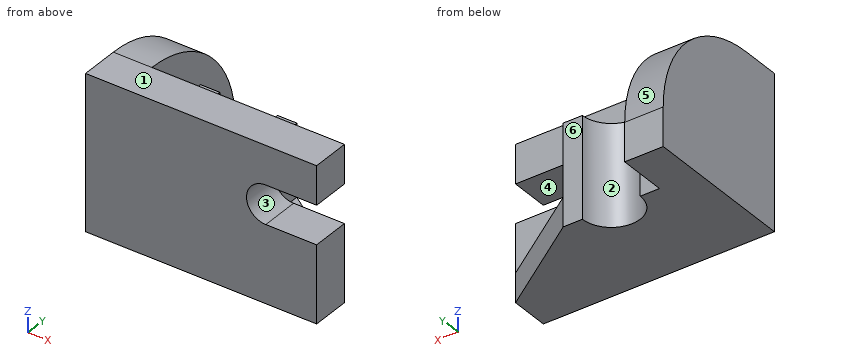
```python
from build123d import *

# Parameters (mm, degrees)
BOSS_EXTRUDE1_DEPTH = 40.64
BOSS_EXTRUDE2_DEPTH = 121.92
BOSS_EXTRUDE3_DEPTH = 71.12
CHAMFER1_SIZE       = 71.12
CHAMFER1_SIZE2      = 101.6
FILLET1_R           = 121.92
CUT_EXTRUDE1_DEPTH  = 106.68


with BuildPart() as part:
    # Sketch1 → Boss-Extrude1 (new body)
    with BuildSketch(Plane(origin=(0, 0, 0), x_dir=(1, 0, 0), z_dir=(0, 1, 0))):
        with BuildLine():
            Line((186.601289805, 121.92), (-57.238710195, 121.92))
            Line((-57.238710195, 121.92), (-57.238710195, -40.64))
            Line((-57.238710195, -40.64), (186.601289805, -40.64))
            Line((186.601289805, -40.64), (186.601289805, 0))
            Line((186.601289805, 0), (132.948481924, 0))
            ThreePointArc((132.948481924, 0), (112.628481924, 20.32), (132.948481924, 40.64))
            Line((132.948481924, 40.64), (186.601289805, 40.64))
            Line((186.601289805, 40.64), (186.601289805, 121.92))
        make_face()
    extrude(amount=BOSS_EXTRUDE1_DEPTH)

    # Sketch2 → Boss-Extrude2 (add)
    with BuildSketch(Plane(origin=(0, 40.64, 0), x_dir=(1, 0, 0), z_dir=(0, 1, 0))):
        Polygon((-16.598710195, 15.24), (-16.598710195, 121.92), (-57.238710195, 121.92), (-57.238710195, -40.64), (-16.598710195, -40.64), align=None)
    extrude(amount=BOSS_EXTRUDE2_DEPTH)

    # Sketch2<4> → Boss-Extrude3 (add)
    with BuildSketch(Plane(origin=(0, 40.64, 0), x_dir=(1, 0, 0), z_dir=(0, 1, 0))):
        Polygon((-16.598710195, 15.24), (85.001289805, 15.24), (85.001289805, 91.44), (186.601289805, 91.44), (186.601289805, 121.92), (-16.598710195, 121.92), align=None)
    extrude(amount=BOSS_EXTRUDE3_DEPTH)

    # Chamfer1
    chamfer1_edges = [part.edges().sort_by_distance(p)[0] for p in [
        (186.601289805, 111.76, -106.68),
    ]]
    chamfer1_side = [part.faces().sort_by_distance(p)[0] for p in [
        (186.601289805, 20.32, -42.021909404),
    ]]
    chamfer(chamfer1_edges, length=CHAMFER1_SIZE, length2=CHAMFER1_SIZE2, reference=chamfer1_side[0])

    # Fillet1
    fillet1_edges = [part.edges().sort_by_distance(p)[0] for p in [
        (-36.918710195, 162.56, 40.64),
    ]]
    fillet(fillet1_edges, radius=FILLET1_R)

    # Sketch3 → Cut-Extrude1 (cut)
    with BuildSketch(Plane.XY.offset(-15.24)):
        with BuildLine():
            Line((64.681289805, 111.76), (3.721289805, 111.76))
            ThreePointArc((3.721289805, 111.76), (34.201289805, 81.28), (64.681289805, 111.76))
        make_face()
    extrude(amount=-CUT_EXTRUDE1_DEPTH, mode=Mode.SUBTRACT)


solid = part.part
```
Can you work these out from the model? Positions are in its coordinate system, mm. Face numbers are marked on the shaded views. A direction names the side the tool comes from. Round coordinates to 2 decimals unless told otherwise and drop trailing zeros. Loops run counter-clockwise (first coordinate to the right, second up) from the corner with the lowest first, then second, coordinate; pieces in that order, holes last. Notation, with made-up numbers: (-13.5, 19) -> (6.5, 19) arc R25 ccw to (6.5, 33) -> close; hole circle Ø7 at (14, -5.75). An arc over 180 degrees is marked (long way). One line per item, written item: value. Start each with the question number.
1. If we section it at C-C, the plane x = 118.5: Write out the boundary of the cut face in (y, z).
2. If we section it at B-B, the plane y = 108: Write out the boundary of the cut face in (x, z).
3. For the marked faces 4, 5 and 6, which set-ups out of +Z, -Z, +X, -X, +Y, -Y let a thin tool reach every point of the face, with its end or its side?
4. For pin 1 (12 mm diameter, centred on y = 50, z = -20, fed in from +X); pin 2 (6 mm diameter, centred on x = -6.5, z = -70, fed in from +Y); pin 3 (21.5 mm diameter, centred on x = 53, y = 59, fed in from +Z), each with a flat end and sliding along its axis, tell me the tip position at first contact or that it passes through.
5. If we section it at A-A, the plane z = -94.5: Write out the boundary of the cut face in (x, y).
6. If we mould it in two halves opening along Z, with no side actions, what happens to the marked faces 1, 2 and 3? For each: pulls with the +Z half, pulls with the -Z half, needs draft (parallel to the pull), parting line crosses it, or undercut.
7. If we section it at D-D, the plane y = 68.5: Write out the boundary of the cut face in (x, z), then the cut area to 3 significant figures.
8. If I drill on probe 1 along Y at (x, z) = (11.5, -2); probe 2 along X at (y, z) = (56, -32); probe 3 along X at (y, z) = (147, -35.5), over which ranges is the centre line in solid material (lowest first)?
Calculated:
1. outline: (0, -121.92) -> (88.31, -121.92) -> (88.31, -91.44) -> (40.64, -91.44) -> (40.64, -34.61) -> (0, -34.61) -> close; (0, -6.03) -> (40.64, -6.03) -> (40.64, 40.64) -> (0, 40.64) -> close
2. outline: (-57.24, -121.92) -> (3.95, -121.92) -> (3.95, -15.24) -> (-16.6, -15.24) -> (-16.6, 20.34) -> (-57.24, 20.34) -> close; (64.45, -121.92) -> (90.37, -121.92) -> (90.37, -91.44) -> (85, -91.44) -> (85, -15.24) -> (64.45, -15.24) -> close
3. face 4: +X, +Y, -Y
3. face 5: +Z, +X, -X, +Y
3. face 6: +Z, -Z, +X, +Y
4. pin 1: stops at x = 85
4. pin 2: stops at y = 111.76
4. pin 3: stops at z = -15.24
5. outline: (-57.24, 0) -> (186.6, 0) -> (186.6, 40.64) -> (85, 111.76) -> (64.68, 111.76) arc R30.48 cw to (3.72, 111.76) -> (-16.6, 111.76) -> (-16.6, 162.56) -> (-57.24, 162.56) -> close
6. face 1: pulls with the +Z half
6. face 2: needs draft
6. face 3: undercut
7. outline: (-57.24, -121.92) -> (146.8, -121.92) -> (146.8, -91.44) -> (85, -91.44) -> (85, -15.24) -> (-16.6, -15.24) -> (-16.6, 37.41) -> (-57.24, 37.41) -> close
7. area: 19,200 mm²
8. probe 1: y = 0 to 40.64
8. probe 2: x = -57.24 to 85
8. probe 3: x = -57.24 to -16.6
